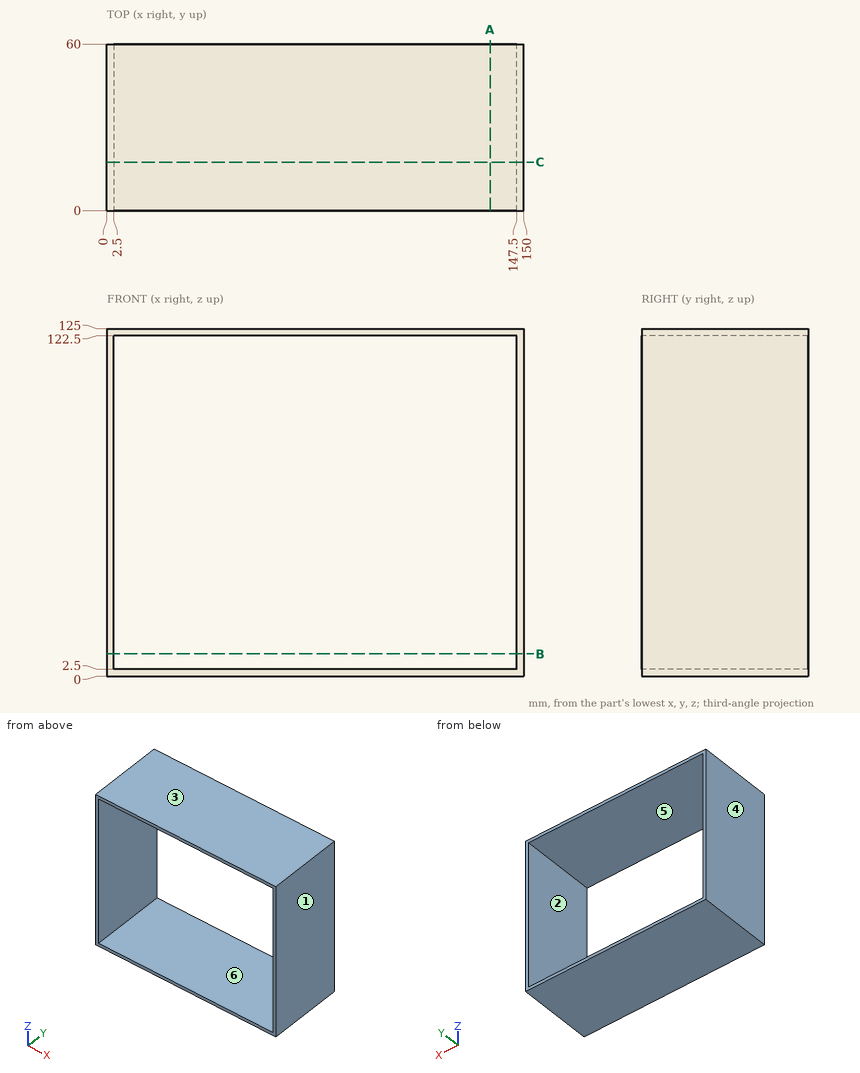
Print and shaded views of the part. All mm, measured from the part's lowest x, y and z. A direction names the side the tool comes from. Coordinates: 2 decimals unless noted, no trailing zeros. Order: outer loops, then holes, each group sorted by start corner. A loop starts at its lowest first (then second) coordinate and runs counter-clockwise, first axis right, second up. Notation, with made-up numbers: (-15.75, -17) -> (4.25, -17) arc R23 ccw to (4.25, 21) -> close; hole circle Ø11 at (59, 81). An arc over 180 degrees is marked (long way). Use one line per item in the form item = value. Start each with the question number.
1) Band-saw the part on A-A on x = 138. Give the cut face in (y, z), then the cut area to 3 significant figures.
2) Pull direction X, two halves, no side cores. Call the marked faces 3, 4, 5 and 6: +X half, -X half, draft (parallel to the pull), parting line (faces both ways), or undercut.
3) Drop a flat-ended pin along its axis: pin 1 (1 mm diameter, centred on x = 94, y = 29, fed in from -Z). Give the stop position or say it passes through.
4) Drill centre lines: L1, parallel to X at y = 55.5, z = 111; L2, parallel to Z at x = 19.5, y = 21. Where is each one in solid material? Low to high. Write a range as [from, to].
5) Band-saw the part on C-C on y = 17.5. Give the cut face in (x, z), then the cut area to 3 significant figures.
6) Tool access for the marked faces 1 and 2: list every direction of +Z, -Z, +X, -X, +Y, -Y with a clear straight run to the whole face (end or side of a thin tool).
7) Band-saw the part on B-B on z = 8. Give the cut face in (x, y).
Entries:
q1.outline = (0, 0) -> (60, 0) -> (60, 2.5) -> (0, 2.5) -> close; (0, 122.5) -> (60, 122.5) -> (60, 125) -> (0, 125) -> close
q1.area = 300 mm2
q2.face_3 = draft
q2.face_4 = -X half
q2.face_5 = undercut
q2.face_6 = undercut
q3.pin_1 = 0
q4.L1 = [0, 2.5], [147.5, 150]
q4.L2 = [0, 2.5], [122.5, 125]
q5.outline = (0, 0) -> (150, 0) -> (150, 125) -> (0, 125) -> close; hole (2.5, 2.5) -> (147.5, 2.5) -> (147.5, 122.5) -> (2.5, 122.5) -> close
q5.area = 1,350 mm2
q6.face_1 = +Z, -Z, +X, +Y, -Y
q6.face_2 = +Y, -Y
q7.outline = (0, 0) -> (2.5, 0) -> (2.5, 60) -> (0, 60) -> close; (147.5, 0) -> (150, 0) -> (150, 60) -> (147.5, 60) -> close
